Print and shaded views of the part. All mm, measured from the part's lowest x, y and z. Round coordinates to 2 decimals unless told otherwise and drop trailing zeros. Loops run counter-clockwise (first coordinate to the right, second up) from the corner with the lowest first, then second, coordinate; pieces in that order, holes last. Notation, with made-up numbers: (63.5, 64) -> (84.5, 64) arc R23 cw to (84.5, 102) -> close; hole circle Ø9 at (39.25, 47.5). An arc over 180 degrees is marked (long way). Answer as CSV lines item,"result".
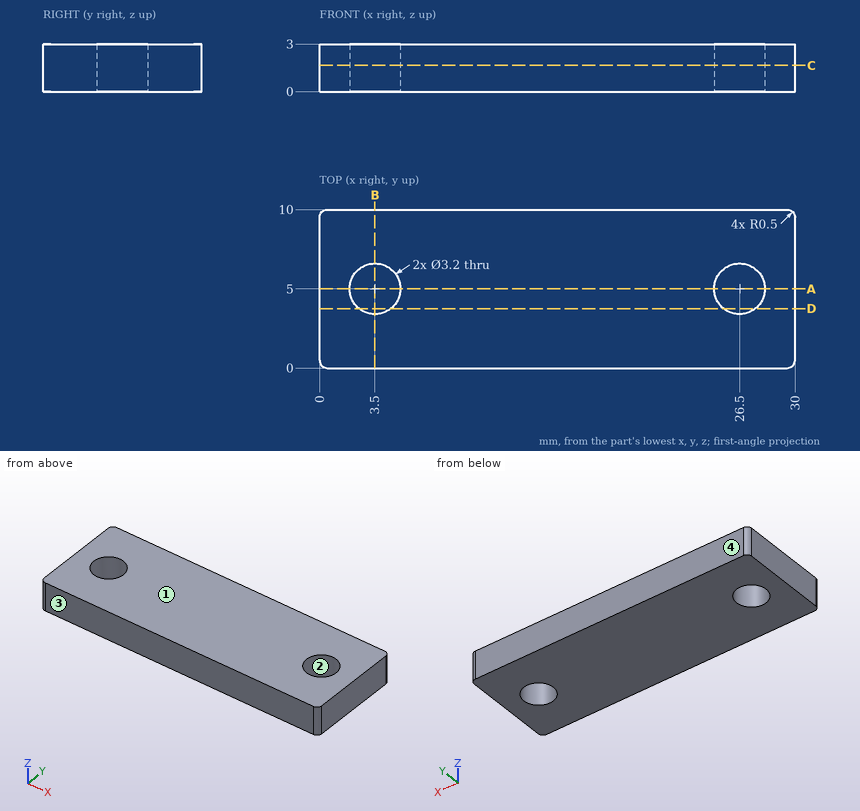
Q1. Slice it at D-D, the plane y = 3.75. Give the cut face in (x, z), and give its area (3 significant figures).
Results:
outline,"(0, 0) -> (2.5, 0) -> (2.5, 3) -> (0, 3) -> close; (4.5, 0) -> (25.5, 0) -> (25.5, 3) -> (4.5, 3) -> close; (27.5, 0) -> (30, 0) -> (30, 3) -> (27.5, 3) -> close"
area,"78.0 mm2"
Q2. Slice it at B-B, the plane x = 3.5. Give the cut face in (y, z).
Results:
outline,"(0, 0) -> (3.4, 0) -> (3.4, 3) -> (0, 3) -> close; (6.6, 0) -> (10, 0) -> (10, 3) -> (6.6, 3) -> close"
Q3. Drop a flat-ended pin along its axis: pin 1 Ø3.5 at (x, y) = (3.5, 5) entering from +Z. Give the stop position or say it passes through.
Results:
pin 1,"z = 3"
Q4. Slice it at A-A, the plane y = 5. Give the cut face in (x, z).
Results:
outline,"(0, 0) -> (1.9, 0) -> (1.9, 3) -> (0, 3) -> close; (5.1, 0) -> (24.9, 0) -> (24.9, 3) -> (5.1, 3) -> close; (28.1, 0) -> (30, 0) -> (30, 3) -> (28.1, 3) -> close"
Q5. Two-plate mould, pull along Y, no slides. Class the marked faces 1, 2, 3 and 4: pulls with the +Y half, pulls with the -Y half, needs draft (parallel to the pull), parting line crosses it, or undercut.
Results:
face 1,"needs draft"
face 2,"undercut"
face 3,"pulls with the -Y half"
face 4,"pulls with the +Y half"
Q6. Probe L1, parallel to Y at x = 3.5, z = 1.95; L2, parallel to X at y = 4.75, z = 0.5; L3, parallel to Y at x = 27.75, z = 2.25. List the from-to ranges inside material, lowest first. Write a range as [from, to].
Results:
L1,"[0, 3.4], [6.6, 10]"
L2,"[0, 1.92], [5.08, 24.92], [28.08, 30]"
L3,"[0, 4], [6, 10]"
Q7. Slice it at C-C, the plane z = 1.65. Give the cut face in (x, y).
Results:
outline,"(0, 0.5) arc R0.5 ccw to (0.5, 0) -> (29.5, 0) arc R0.5 ccw to (30, 0.5) -> (30, 9.5) arc R0.5 ccw to (29.5, 10) -> (0.5, 10) arc R0.5 ccw to (0, 9.5) -> close; hole circle Ø3.2 at (3.5, 5); hole circle Ø3.2 at (26.5, 5)"
